Here's the drawing with two shaded views (mm, measured from the low corner). I have some questions. Round coordinates to 2 decimals unless told otherwise and drop trailing zeros. Order: outer loops, then holes, each group sorted by start corner. A loop starts at its lowest first (then second) coordinate and runs counter-clockwise, first axis right, second up. Notation, with made-up numbers: (-34.5, 36.5) -> (24.5, 36.5) arc R11 cw to (24.5, 51.5) -> close; hole circle Ø10 at (23.25, -30.75). An arc over 180 degrees is marked (long way). One line per question, with ' | ' between items.
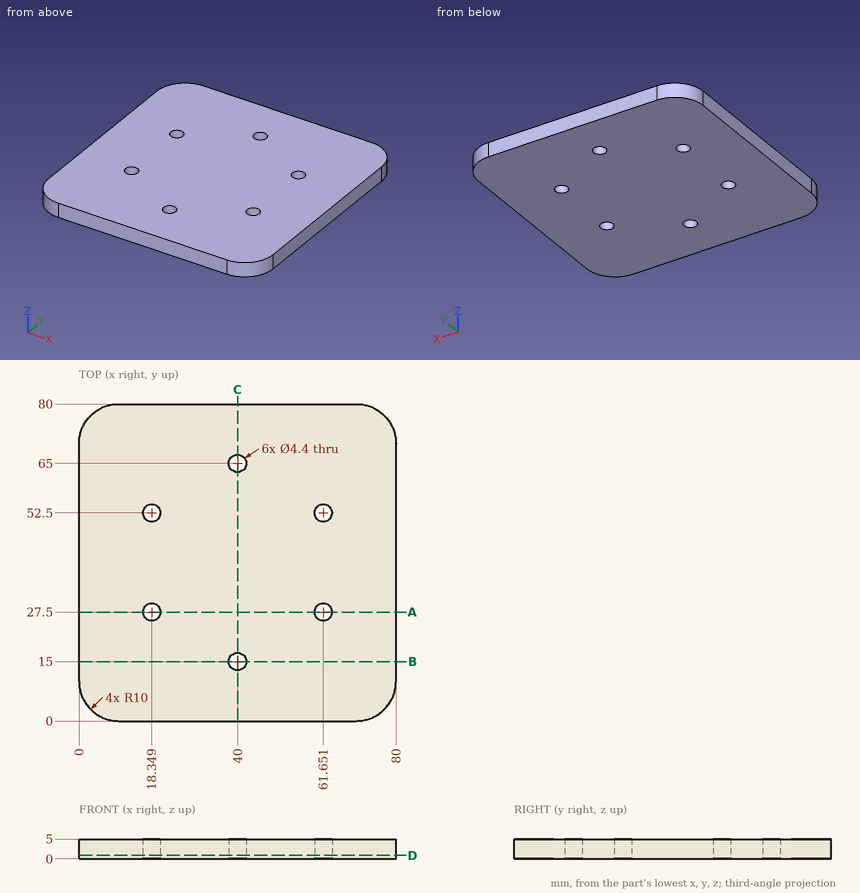
1. I need wall thicknesses on probe 1 along Y at (x, z) = (40, 1.45); probe 2 along Y at (x, z) = (19.5, 3) (1 decimal); probe 3 along X at (y, z) = (29, 1.1). Which ranges of each line are inside material? Lowest first, please.
From the geometry:
probe 1: y = 0 to 12.8, 17.2 to 62.8, 67.2 to 80 | probe 2: y = 0 to 25.6, 29.4 to 50.6, 54.4 to 80 | probe 3: x = 0 to 16.74, 19.96 to 60.04, 63.26 to 80
2. I want a section at D-D on z = 0.85. List the corners of the cut face in (x, y) for me, and give its area (3 significant figures).
From the geometry:
outline: (0, 10) arc R10 ccw to (10, 0) -> (70, 0) arc R10 ccw to (80, 10) -> (80, 70) arc R10 ccw to (70, 80) -> (10, 80) arc R10 ccw to (0, 70) -> close; hole circle Ø4.4 at (18.35, 27.5); hole circle Ø4.4 at (18.35, 52.5); hole circle Ø4.4 at (40, 15); hole circle Ø4.4 at (40, 65); hole circle Ø4.4 at (61.65, 27.5); hole circle Ø4.4 at (61.65, 52.5) | area: 6,220 mm²
3. I want a section at C-C on x = 40. List the corners of the cut face in (y, z) for me.
From the geometry:
outline: (0, 0) -> (12.8, 0) -> (12.8, 5) -> (0, 5) -> close; (17.2, 0) -> (62.8, 0) -> (62.8, 5) -> (17.2, 5) -> close; (67.2, 0) -> (80, 0) -> (80, 5) -> (67.2, 5) -> close
4. I want a section at A-A on y = 27.5. List the corners of the cut face in (x, z) for me, and give its area (3 significant figures).
From the geometry:
outline: (0, 0) -> (16.15, 0) -> (16.15, 5) -> (0, 5) -> close; (20.55, 0) -> (59.45, 0) -> (59.45, 5) -> (20.55, 5) -> close; (63.85, 0) -> (80, 0) -> (80, 5) -> (63.85, 5) -> close | area: 356 mm²
5. I want a section at B-B on y = 15. List the corners of the cut face in (x, z) for me, and give its area (3 significant figures).
From the geometry:
outline: (0, 0) -> (37.8, 0) -> (37.8, 5) -> (0, 5) -> close; (42.2, 0) -> (80, 0) -> (80, 5) -> (42.2, 5) -> close | area: 378 mm²
